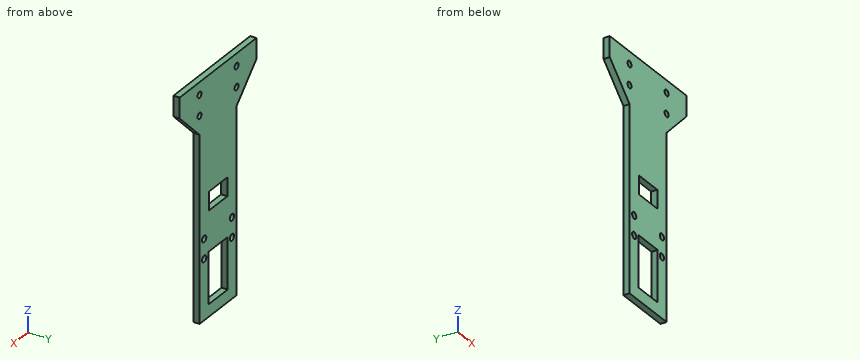
from build123d import *

# Parameters (mm, degrees)
SKETCH1_R           = 1.6
SKETCH1_R_2         = 1.5
SKETCH1_W           = 14
SKETCH1_H           = 9
SKETCH1_W_2         = 14.5
SKETCH1_H_2         = 25
BOSS_EXTRUDE1_DEPTH = 3


with BuildPart() as part:
    # Sketch1 → Boss-Extrude1 (new body)
    with BuildSketch(Plane(origin=(0, 0, 0), x_dir=(1, 0, 0), z_dir=(0, 1, 0))):
        Polygon((0, 0), (0, -90), (15, -105.02919784), (15, -115.02919784), (-43, -115.02919784), (-43, -105.02919784), (-28, -90), (-28, 0), align=None)
        with Locations(Location((-24.5, -38.75, 0), (0, 0, 270))):
            Circle(SKETCH1_R, mode=Mode.SUBTRACT)
        with Locations(Location((-3.5, -38.75, 0), (0, 0, 90))):
            Circle(SKETCH1_R, mode=Mode.SUBTRACT)
        with Locations(Location((-3.5, -29.25, 0), (0, 0, 270))):
            Circle(SKETCH1_R, mode=Mode.SUBTRACT)
        with Locations(Location((-24.5, -29.25, 0), (0, 0, 90))):
            Circle(SKETCH1_R, mode=Mode.SUBTRACT)
        with Locations(Location((-28, -99, 0), (0, 0, 270))):
            Circle(SKETCH1_R_2, mode=Mode.SUBTRACT)
        with Locations(Location((0, -99, 0), (0, 0, 270))):
            Circle(SKETCH1_R_2, mode=Mode.SUBTRACT)
        with Locations(Location((-28, -109, 0), (0, 0, 270))):
            Circle(SKETCH1_R_2, mode=Mode.SUBTRACT)
        with Locations(Location((0, -109, 0), (0, 0, 270))):
            Circle(SKETCH1_R_2, mode=Mode.SUBTRACT)
        with Locations((-14, -55)):
            Rectangle(SKETCH1_W, SKETCH1_H, mode=Mode.SUBTRACT)
        with Locations((-14, -18.5)):
            Rectangle(SKETCH1_W_2, SKETCH1_H_2, mode=Mode.SUBTRACT)
    extrude(amount=BOSS_EXTRUDE1_DEPTH)


solid = part.part
For this review, take the finished solid that the model builds, in its own axes (mm). Round coordinates to 2 decimals unless told otherwise and drop trailing zeros. Loops run counter-clockwise (first coordinate to the right, second up) from the corner with the lowest first, then second, coordinate; pieces in that order, holes last. Notation, with made-up numbers: (-17.75, 87.5) - (27.25, 87.5) arc R30 ccw to (27.25, 109.5) - close; hole circle Ø1 at (-7.75, 16.5). An arc over 180 degrees is marked (long way). Use one line per item in the form item = value.
1) We need section B-B on z = 29.25. Write out the cut boundary in (x, y).
Solutions:
outline = (-28, 0) - (-26.1, 0) - (-26.1, 3) - (-28, 3) - close; (-22.9, 0) - (-21.25, 0) - (-21.25, 3) - (-22.9, 3) - close; (-6.75, 0) - (-5.1, 0) - (-5.1, 3) - (-6.75, 3) - close; (-1.9, 0) - (0, 0) - (0, 3) - (-1.9, 3) - close
2) Clearance check with a flat-ended pin moving along its axis: P1, Ø0.9, axis at y = 2, z = 53, coming from the -X side. State where the tip first meets the part, or that it passes through.
Solutions:
P1 = -28
3) We need section D-D on y = 1. State how many separate pieces and enclosed holes the cut face has, then the cut area to 3 significant figures.
Solutions:
separate_pieces = 1
enclosed_holes = 10
area = 3,200 mm2
4) We need section A-A on x = -10.5. Write out the cut boundary in (y, z).
Solutions:
outline = (0, 0) - (3, 0) - (3, 6) - (0, 6) - close; (0, 31) - (3, 31) - (3, 50.5) - (0, 50.5) - close; (0, 59.5) - (3, 59.5) - (3, 115.03) - (0, 115.03) - close
5) Wall thickness on probe 1 along X at (y, z) = (2, 29.25); probe 2 along Z at (x, y) = (-8.5, 0.2); probe 3 along Z at (x, y) = (-0.5, 2.05): over which ranges is each line inside the solid? List them lowest first.
Solutions:
probe_1 = -28 to -26.1, -22.9 to -21.25, -6.75 to -5.1, -1.9 to 0
probe_2 = 0 to 6, 31 to 50.5, 59.5 to 115.03
probe_3 = 0 to 97.59, 100.41 to 107.59, 110.41 to 115.03
6) We need section C-C on z = 53. Write out the cut boundary in (x, y), then the cut area to 3 significant figures.
Solutions:
outline = (-28, 0) - (-21, 0) - (-21, 3) - (-28, 3) - close; (-7, 0) - (0, 0) - (0, 3) - (-7, 3) - close
area = 42.0 mm2
